CAD build for the part. Positions are in the model's coordinates, mm. Face numbers are marked on the shaded views. Give positions to 0.01 mm unless a question says otherwise; leave off trailing zeros. Loops run counter-clockwise (first coordinate to the right, second up) from the corner with the lowest first, then second, coordinate; pieces in that order, holes last. Notation, with made-up numbers: M 77.25,40.25 L 129.25,40.25 A12 cw 129.25,46.25 Z; hole C 35,61.5 d5. An arc over 180 degrees is marked long. One line per question, with ' | ' between items.
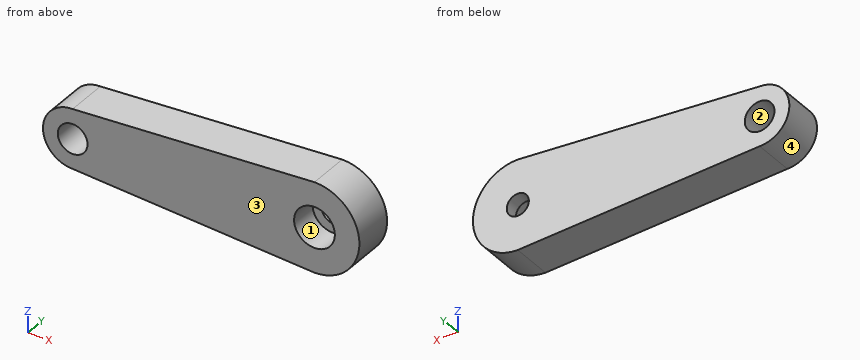
```python
from build123d import *

# Parameters (mm, degrees)
BOSS_EXTRUDE1_DEPTH = 6
SKETCH2_R           = 2.15
CUT_EXTRUDE1_DEPTH  = 6
SKETCH3_R           = 2.95
CUT_EXTRUDE2_DEPTH  = 4
SKETCH4_R           = 1.6
CUT_EXTRUDE3_DEPTH  = 11


with BuildPart() as part:
    # Sketch1 → Boss-Extrude1 (new body)
    with BuildSketch(Plane(origin=(0, 0, 0), x_dir=(1, 0, 0), z_dir=(0, 1, 0))):
        with BuildLine():
            Line((-35, 4.3), (0, 6.5))
            ThreePointArc((0, 6.5), (6.5, 0), (0, -6.5))
            Line((0, -6.5), (-35, -4.3))
            ThreePointArc((-35, -4.3), (-39.3, 0), (-35, 4.3))
        make_face()
    extrude(amount=BOSS_EXTRUDE1_DEPTH)

    # Sketch2 → Cut-Extrude1 (cut)
    with BuildSketch(Plane(origin=(0, 0, 0), x_dir=(1, 0, 0), z_dir=(0, 1, 0))):
        with Locations(Location((-35, 0, 0), (0, 0, 270))):
            Circle(SKETCH2_R)
    extrude(amount=CUT_EXTRUDE1_DEPTH, mode=Mode.SUBTRACT)

    # Sketch3 → Cut-Extrude2 (cut)
    with BuildSketch(Plane(origin=(0, 0, 0), x_dir=(1, 0, 0), z_dir=(0, 1, 0))):
        with Locations(Location((0, 0, 0), (0, 0, 270))):
            Circle(SKETCH3_R)
    extrude(amount=CUT_EXTRUDE2_DEPTH, mode=Mode.SUBTRACT)

    # Sketch4 → Cut-Extrude3 (cut)
    with BuildSketch(Plane(origin=(0, 0, 0), x_dir=(1, 0, 0), z_dir=(0, 1, 0))):
        with Locations(Location((0, 0, 0), (0, 0, 270))):
            Circle(SKETCH4_R)
    extrude(amount=CUT_EXTRUDE3_DEPTH, mode=Mode.SUBTRACT)


solid = part.part
```
Item 1: Drop flat-ended pins along their axis: P1, Ø1, axis at x = -12.5, y = 1.5, coming from the +Z side; P2, Ø3.5, axis at x = 0, z = 0, coming from the -Y side; P3, Ø1.5, axis at x = -18, y = 3.5, coming from the +Z side. Give the stop position or say it passes through.
Conclusion:
P1: z = 5.75 | P2: y = 4 | P3: z = 5.42
Item 2: Saw through at A-A on z = 0. Give the cut face in (x, y), and give its area (3 significant figures).
Conclusion:
outline: M -39.3,0 L -37.15,0 L -37.15,6 L -39.3,6 Z; M -32.85,0 L -2.95,0 L -2.95,4 L -1.6,4 L -1.6,6 L -32.85,6 Z; M 1.6,4 L 2.95,4 L 2.95,0 L 6.5,0 L 6.5,6 L 1.6,6 Z | area: 219 mm²
Item 3: Saw through at B-B on y = 4.75. Give the cut face in (x, z).
Conclusion:
outline: M -35,-4.3 L 0,-6.5 A6.5 ccw 0,6.5 L -35,4.3 A4.3 ccw Z; hole C -35,0 d4.3; hole C 0,0 d3.2
Item 4: Mould opens along X. For the marked faces 1, 2, 3 and 4 say: pulls with the +X half, pulls with the -X half, needs draft (parallel to the pull), parting line crosses it, or undercut.
Conclusion:
face 1: undercut | face 2: undercut | face 3: needs draft | face 4: pulls with the -X half
Item 5: Drill centre lines: line 1 along X through (y, z) = (2.45, 0); line 2 along X through (y, z) = (5.2, 0); line 3 along Z through (x, y) = (0.5, 1.5). Where is each one in solid material? Low to high. Write a range as [from, to].
Conclusion:
line 1: [-39.3, -37.15], [-32.85, -2.95], [2.95, 6.5] | line 2: [-39.3, -37.15], [-32.85, -1.6], [1.6, 6.5] | line 3: [-6.48, -2.91], [2.91, 6.48]
Item 6: Saw through at D-D on x = -7. Give the cut face in (y, z), and give its area (3 significant figures).
Conclusion:
outline: M 0,-6.06 L 6,-6.06 L 6,6.06 L 0,6.06 Z | area: 72.7 mm²
Item 7: Saw through at C-C on x = 1. Give the cut face in (y, z).
Conclusion:
outline: M 0,-6.42 L 6,-6.42 L 6,-1.25 L 4,-1.25 L 4,-2.78 L 0,-2.78 Z; M 0,2.78 L 4,2.78 L 4,1.25 L 6,1.25 L 6,6.42 L 0,6.42 Z
